Input: part model. Units: mm. Frame: model coordinates. Round coordinates to 2 decimals unless told otherwise and drop trailing zeros. Order: outer loops, then holes, each group sorted by start corner. A loop starts at its lowest first (then second) coordinate and runs counter-clockwise, first axis right, second up. Notation, with made-up numbers: (44.25, -3) -> (75.25, -3) arc R11 ccw to (75.25, 5) -> close; hole circle Ø1 at (18, -19). An arc over 180 degrees is marked (long way). Use a Markdown table: item, result.
from build123d import *

# Parameters (mm, degrees)
SKETCH1_R               = 9.825
SKETCH1_R_2             = 2.505
BOSS_EXTRUDE1_DEPTH     = 25
SKETCH2_R               = 4
CUT_EXTRUDE1_DEPTH      = 13.5
CUT_EXTRUDE2_DEPTH      = 13.5
CUT_EXTRUDE2_DEPTH_BACK = 13.5
CUT_EXTRUDE3_DEPTH      = 13.5


with BuildPart() as part:
    # Sketch1 → Boss-Extrude1 (new body)
    with BuildSketch(Plane(origin=(0, 0, 0), x_dir=(1, 0, 0), z_dir=(0, 1, 0))):
        with Locations(Location((0, 0, 0), (0, 0, 270))):
            Circle(SKETCH1_R)
        with Locations(Location((0, 0, 0), (0, 0, 270))):
            Circle(SKETCH1_R_2, mode=Mode.SUBTRACT)
    extrude(amount=BOSS_EXTRUDE1_DEPTH)

    # Sketch2 → Cut-Extrude1 (cut)
    with BuildSketch(Plane(origin=(0, 25, 0), x_dir=(1, 0, 0), z_dir=(0, 1, 0))):
        with Locations(Location((0, 0, 0), (0, 0, 270))):
            Circle(SKETCH2_R)
    extrude(amount=-CUT_EXTRUDE1_DEPTH, mode=Mode.SUBTRACT)

    # Sketch3 → Cut-Extrude2 (cut, two sides: drawn at the far end of the back side and taken through both)
    with BuildSketch(Plane.XY.offset(-CUT_EXTRUDE2_DEPTH_BACK)):
        Polygon((-9.825, 12.5), (-9.825, 12.95), (0, 12.95), (0, 12.5), (0, 12.05), (-9.825, 12.05), align=None)
    extrude(amount=CUT_EXTRUDE2_DEPTH + CUT_EXTRUDE2_DEPTH_BACK, mode=Mode.SUBTRACT)

    # Sketch5 → Cut-Extrude3 (cut)
    with BuildSketch(Plane.XY):
        Polygon((0, 0), (-0.45, 0), (-0.45, 25), (0, 25), (0.45, 25), (0.45, 0), align=None)
    extrude(amount=-CUT_EXTRUDE3_DEPTH, mode=Mode.SUBTRACT)


solid = part.part
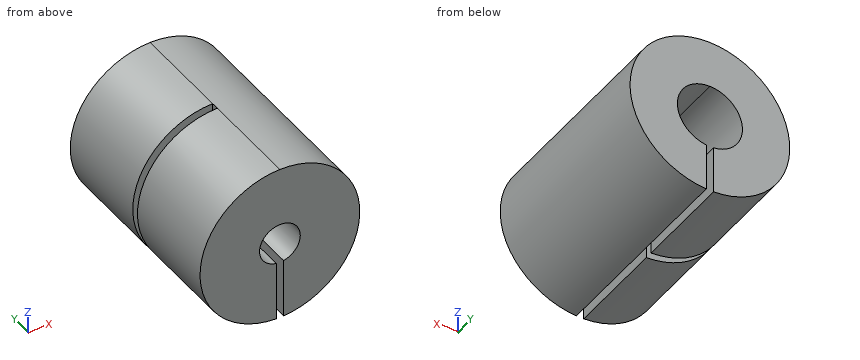
1) Cut plane C-C on x = -1.75. Return loops of the section in (y, z), and give its area (3 significant figures).
Answer key:
| item | result |
|---|---|
| outline | (0, -9.67) -> (12.05, -9.67) -> (12.05, -3.6) -> (11.5, -3.6) -> (11.5, -1.79) -> (0, -1.79) -> close; (0, 1.79) -> (11.5, 1.79) -> (11.5, 3.6) -> (12.05, 3.6) -> (12.05, 9.67) -> (0, 9.67) -> close; (12.95, -9.67) -> (25, -9.67) -> (25, -3.6) -> (12.95, -3.6) -> close; (12.95, 3.6) -> (25, 3.6) -> (25, 9.67) -> (12.95, 9.67) -> close |
| area | 334 mm^2 |
2) Cut plane A-A on x = -7.75. Return loops of the section in (y, z).
Answer key:
| item | result |
|---|---|
| outline | (0, -6.04) -> (12.05, -6.04) -> (12.05, 6.04) -> (0, 6.04) -> close; (12.95, -6.04) -> (25, -6.04) -> (25, 6.04) -> (12.95, 6.04) -> close |
3) Ray query, probe 1 along Y at (x, z) = (-5, -1); probe 2 along Y at (x, z) = (2, 2); probe 3 along X at (y, z) = (7.5, 0) (3 decimals). Return the intervals inside material, ascending.
Answer key:
| item | result |
|---|---|
| probe 1 | y = 0 to 12.05, 12.95 to 25 |
| probe 2 | y = 0 to 11.5 |
| probe 3 | x = -9.825 to -2.505, 2.505 to 9.825 |
4) Contact query for flat-ended pins moving along their axis: P1, Ø6, axis at y = 16.5, z = -5.5, coming from the -X side; P2, Ø9, axis at x = 1.5, z = 0, coming from the +Y side; P3, Ø8, axis at y = 4, z = -7.5, coming from the +X side; P4, Ø2, axis at x = 2.5, y = 15.5, coming from the -Z side. Output: stop coordinate, or through.
Answer key:
| item | result |
|---|---|
| P1 | stops at x = -9.5 |
| P2 | stops at y = 25 |
| P3 | stops at x = 9.18 |
| P4 | stops at z = -9.71 |
5) Cut plane B-B on z = 0. Return loops of the section in (x, y) (3 decimals), and give its area (3 significant figures).
Answer key:
| item | result |
|---|---|
| outline | (-9.825, 0) -> (-2.505, 0) -> (-2.505, 11.5) -> (-4, 11.5) -> (-4, 12.05) -> (-9.825, 12.05) -> close; (-9.825, 12.95) -> (-4, 12.95) -> (-4, 25) -> (-9.825, 25) -> close; (2.505, 0) -> (9.825, 0) -> (9.825, 25) -> (4, 25) -> (4, 11.5) -> (2.505, 11.5) -> close |
| area | 320 mm^2 |
6) Cut plane D-D on z = -3.25. Return loops of the section in (x, y), and give its area (3 significant figures).
Answer key:
| item | result |
|---|---|
| outline | (-9.27, 0) -> (-0.45, 0) -> (-0.45, 11.5) -> (-2.33, 11.5) -> (-2.33, 12.05) -> (-9.27, 12.05) -> close; (-9.27, 12.95) -> (-2.33, 12.95) -> (-2.33, 25) -> (-9.27, 25) -> close; (0.45, 0) -> (9.27, 0) -> (9.27, 25) -> (2.33, 25) -> (2.33, 11.5) -> (0.45, 11.5) -> close |
| area | 384 mm^2 |
